```python
from build123d import *

# Parameters (mm, degrees)
F1_DEPTH  = 18
F3_D      = 3.2
F3_DEPTH  = 15
F4_W      = 6
F4_H      = 6
F5_DEPTH  = 10
F6_W      = 6
F6_H      = 6
F7_DEPTH  = 10
F9_D      = 3.2
F9_DEPTH  = 6
F11_D     = 3.2
F11_DEPTH = 6


with BuildPart() as f1:
    # F0 (on Top) → F1 (new body)
    with BuildSketch(Plane.XY):
        with BuildLine():
            Line((3, 13.278079), (-6.7, 13.278079))
            Line((-6.7, 13.278079), (-6.7, 10.278079))
            Line((-6.7, 10.278079), (0.622289, 10.278079))
            ThreePointArc((0.622289, 10.278079), (11.5, 2.620549), (22.377711, 10.278079))
            Line((22.377711, 10.278079), (23, 10.278079))
            Line((23, 10.278079), (29.7, 10.278079))
            Line((29.7, 10.278079), (29.7, 17.778079))
            Line((29.7, 17.778079), (22.406277, 17.778079))
            ThreePointArc((22.406277, 17.778079), (11.5, 25.549511), (0.593723, 17.778079))
            Line((0.593723, 17.778079), (-6.7, 17.778079))
            Line((-6.7, 17.778079), (-6.7, 14.778079))
            Line((-6.7, 14.778079), (3, 14.778079))
            ThreePointArc((3, 14.778079), (11.5, 22.528734), (20, 14.778079))
            Line((20, 14.778079), (25.6, 14.778079))
            Line((25.6, 14.778079), (25.6, 13.278079))
            Line((25.6, 13.278079), (23, 13.278079))
            Line((23, 13.278079), (20, 13.278079))
            ThreePointArc((20, 13.278079), (11.5, 5.523889), (3, 13.278079))
        make_face()
    extrude(amount=F1_DEPTH)

    # F3
    with Locations(Plane.XZ.offset(-10.278079)):
        with Locations((-3.038855, 9)):
            Hole(F3_D / 2, depth=F3_DEPTH)

    # F4 (on face) → F5 (join)
    with BuildSketch(Plane.XZ.offset(-10.278079)):
        with Locations((26.7, 3)):
            Rectangle(F4_W, F4_H)
    extrude(amount=F5_DEPTH)

    # F6 (on face) → F7 (join)
    with BuildSketch(Plane.XZ.offset(-10.278079)):
        with Locations((-3.7, 3)):
            Rectangle(F6_W, F6_H)
    extrude(amount=F7_DEPTH)

    # F9
    with Locations(Plane.YZ.offset(29.7)):
        with Locations((3.748374, 3)):
            Hole(F9_D / 2, depth=F9_DEPTH)

    # F11
    with Locations(Plane(origin=(-6.7, 0, 0), x_dir=(0, -1, 0), z_dir=(-1, 0, 0))):
        with Locations((-3.278079, 3)):
            Hole(F11_D / 2, depth=F11_DEPTH)


solid = f1.part
```
Source: CAD feature listing. Evaluate the final solid. Frame: model axes, mm. A direction names the side the tool comes from. Round coordinates to 2 decimals unless told otherwise and drop trailing zeros. Loops run counter-clockwise (first coordinate to the right, second up) from the corner with the lowest first, then second, coordinate; pieces in that order, holes last. Notation, with made-up numbers: M 60.5,-2.75 L 75.5,-2.75 A23 ccw 75.5,32.25 Z; hole C 15.25,-25 d7. An arc over 180 degrees is marked long. Put each result on its own line as item: value.
(1) Section A-A, the plane x = 23. Return loops of the section in (y, z), and give its area (3 significant figures).
Solutions:
outline: M 10.28,0 L 13.28,0 L 13.28,18 L 10.28,18 Z; M 14.78,0 L 17.78,0 L 17.78,18 L 14.78,18 Z
area: 108 mm²
(2) Section B-B, the plane y = 11.75. Return loops of the section in (x, z), and give its area (3 significant figures).
Solutions:
outline: M -6.7,0 L 3.28,0 L 3.28,18 L -6.7,18 Z; M 19.72,0 L 29.7,0 L 29.7,18 L 19.72,18 Z; hole C -3.04,9 d3.2
area: 351 mm²
(3) Section C-C, the plane z = 3. Return loops of the section in (x, y), and give its area (3 significant figures).
Solutions:
outline: M -6.7,0.28 L -0.7,0.28 L -0.7,1.68 L -6.7,1.68 Z; M -6.7,4.88 L -0.7,4.88 L -0.7,10.28 L 0.62,10.28 A11.55 ccw 22.38,10.28 L 23.7,10.28 L 23.7,5.35 L 29.7,5.35 L 29.7,17.78 L 22.41,17.78 A11.54 ccw 0.59,17.78 L -6.7,17.78 L -6.7,14.78 L 3,14.78 A8.54 cw 20,14.78 L 25.6,14.78 L 25.6,13.28 L 20,13.28 A8.54 cw 3,13.28 L -6.7,13.28 Z; M 23.7,0.28 L 29.7,0.28 L 29.7,2.15 L 23.7,2.15 Z
area: 349 mm²
(4) Section D-D, the plane z = 17. Return loops of the section in (x, y).
Solutions:
outline: M -6.7,10.28 L 0.62,10.28 A11.55 ccw 22.38,10.28 L 29.7,10.28 L 29.7,17.78 L 22.41,17.78 A11.54 ccw 0.59,17.78 L -6.7,17.78 L -6.7,14.78 L 3,14.78 A8.54 cw 20,14.78 L 25.6,14.78 L 25.6,13.28 L 20,13.28 A8.54 cw 3,13.28 L -6.7,13.28 Z
(5) Pull-direction query (Y, two-part tool) for faces 1 (the face through (27, 0.278, 3)), 2 (the face through (23, 13.278, 9)), 3 (the face through (-1, 17.778, 9)); classes: released by +Y, released by -Y, zero draft, split by the parting line, or undercut.
Solutions:
face 1: released by -Y
face 2: undercut
face 3: released by +Y
(6) Access query for faces 4 (the face through (-1, 14.778, 9)), 5 (the face through (26.66, 3.01, 1.58)), 6 (the face through (11.323, 22.527, 8.874)). Directions: +Z, -Z, +X, -X, +Y, -Y. A direction counts if a zero-diameter tool reaches every point of the face in a straight line with its end or side. Return the directions, or none.
Solutions:
face 4: +Z, -Z, -X
face 5: +X
face 6: +Z, -Z
(7) Ray query, line 1 (X direction, y = 11, z = 10.25); line 2 (X direction, y = 14.25, z = 14); line 3 (Z direction, x = 24.5, y = 6.5). Return the intervals inside material, ascending. Write a range as [from, to].
Solutions:
line 1: [-6.7, -4.04], [-2.04, 3.53], [19.47, 29.7]
line 2: [25.6, 29.7]
line 3: [0, 6]
(8) First-contact query: pin 1 (1.9 mm diameter, centred on y = 3.75, z = 3, fed in from -X); pin 2 (3 mm diameter, centred on x = -4, z = 9, fed in from +Y); pin 3 (6 mm diameter, centred on x = 21, z = 3, fed in from +Y); pin 4 (2.5 mm diameter, centred on x = -3.04, z = 9, fed in from +Y). Flat tips, straight axial feed; report the tip coordinate or a pass-through.
Solutions:
pin 1: x = 4.89
pin 2: y = 17.78
pin 3: y = 23.54
pin 4: through
